Here's how the part is built. I have some questions about the finished solid (model axes, mm). Face numbers are marked on the shaded views. Give positions to 0.01 mm unless a question says otherwise; leave off trailing zeros. Loops run counter-clockwise (first coordinate to the right, second up) from the corner with the lowest first, then second, coordinate; pieces in that order, holes last. Notation, with made-up numbers: (78.5, -4.75) - (127.5, -4.75) arc R27 cw to (127.5, 25.25) - close; hole circle Ø3 at (30.5, 40.5). An arc over 180 degrees is marked (long way). Use a Markdown table: item, result.
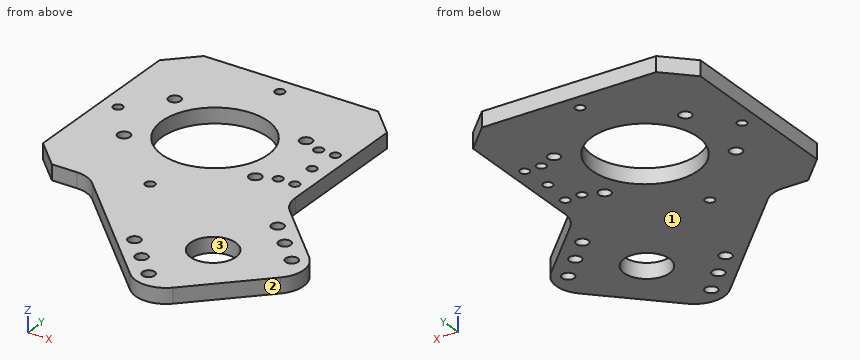
Autodesk Inventor part; units mm, degrees
ref_plane "YZ Plane" through (0, 0, 0) normal (1, 0, 0) x (0, 1, 0)
ref_plane "XZ Plane" through (0, 0, 0) normal (0, 1, 0) x (-1, 0, 0)
ref_plane "XY Plane" through (0, 0, 0) normal (0, 0, 1) x (1, 0, 0)
sketch "Sketch1" plane through (0, 0, 0) normal (0, 0, 1) x (1, 0, 0)
  line L0 (-47.625, -47.625) -> (47.625, -47.625)
  line L1 (47.625, -47.625) -> (47.625, 47.625)
  line L2 (47.625, 47.625) -> (-47.625, 47.625)
  line L3 (-47.625, 47.625) -> (-47.625, -47.625)
  line L4 (-47.625, -47.625) -> (47.625, 47.625) construction
  line L5 (47.625, -47.625) -> (-47.625, 47.625) construction
  point P0 (0, 0)
  dimension "width" = 95.25
  dimension "length" = 95.25
extrude "Extrusion1" add sketch "Sketch1" along normal mid plane 6.35
sketch "Sketch2" plane through (0, 0, 3.175) normal (0, 0, 1) x (1, 0, 0)
  circle A0 centre (0, 0) radius 35
  circle A1 centre (0, 0) radius 60 construction
  circle A2 centre (0, 0) radius 40.64 construction
  point P0 (0, 40.64)
  point P1 (-40.64, 0)
  point P2 (0, -40.64)
  point P3 (40.64, 0)
  dimension "d74" = 81.28
  dimension "d5" = 120
  dimension "d73" = 70
  dimension "d77" = 360
hole "Hole1" at (0, 40.64, 3.175) at (-40.64, 0, 3.175) at (0, -40.64, 3.175) at (40.64, 0, 3.175) direction (0, 0, -1) diameter 3.9624 end through all
sketch "Sketch3" plane through (0, 0, 3.175) normal (0, 0, 1) x (1, 0, 0)
  circle A0 centre (0, 0) radius 31.75 construction
  point P0 (0, 31.75)
  point P1 (-27.4963, 15.875)
  point P2 (-27.4963, -15.875)
  point P3 (0, -31.75)
  point P4 (27.4963, -15.875)
  point P5 (27.4963, 15.875)
  dimension "d17" = 63.5
  dimension "d20" = 360
hole "Hole2" at (-27.4963, 15.875, 3.175) at (-27.4963, -15.875, 3.175) at (27.4963, -15.875, 3.175) at (27.4963, 15.875, 3.175) direction (0, 0, -1) diameter 5.1054 end through all
sketch "Sketch4" plane through (0, 0, 3.175) normal (0, 0, 1) x (1, 0, 0)
  circle A0 centre (0, 0) radius 22.225
  dimension "d30" = 44.45
extrude "Extrusion2" cut sketch "Sketch4" against normal through all
sketch "Sketch5" plane through (0, 0, 3.175) normal (0, 0, 1) x (1, 0, 0)
  circle A0 centre (0, 0) radius 64 construction
  circle A1 centre (45.021, -68.5355) radius 18 construction
  line L0 (95.821, 47.9105) -> (95.821, -47.9105) construction
  line L1 (54.0013, -41.5947) -> (18.0802, -77.5157) construction
  line L2 (18.0802, -77.5157) -> (27.0605, -86.496) construction
  line L3 (36.0407, -59.5552) -> (45.021, -68.5355) construction
  line L4 (-47.625, -47.625) -> (47.625, -47.625) construction
  line L5 (-20.7907, -47.625) -> (39.7884, -108.2042)
  line L6 (39.7884, -108.2042) -> (84.6897, -63.3029)
  line L7 (84.6897, -63.3029) -> (47.625, -26.2382)
  line L8 (47.625, -47.625) -> (47.625, 47.625) construction
  line L9 (-20.7907, -47.625) -> (47.625, -47.625)
  line L10 (47.625, -47.625) -> (47.625, -26.2382)
  circle A2 centre (45.021, -68.5355) radius 9.525
  point P0 (95.821, 0)
  point P1 (27.0605, -86.496)
  point P2 (36.0407, -95.4762)
  point P3 (62.9815, -50.5749)
  point P4 (62.9815, -50.5749)
  point P5 (71.9618, -59.5552)
  point P6 (-22.225, -47.625)
  dimension "d33" = 128
  dimension "d34" = 36
  dimension "d35" = 95.821
  dimension "d36" = 95.821
  dimension "d37" = 50.8
  dimension "d38" = 12.7
  dimension "d39" = 12.7
  dimension "d42" = 12.7
  dimension "d47" = 45
  dimension "d48" = 50.8
  dimension "d49" = 6.35
  dimension "d50" = 24.35
  dimension "d51" = 6.35
  dimension "d55" = 19.05
  dimension "d64" = 45
extrude "Extrusion3" add sketch "Sketch5" against normal up to surface (6.35 mm away)
hole "Hole3" at (18.0802, -77.5157, 3.175) at (27.0605, -86.496, 3.175) at (36.0407, -95.4762, 3.175) at (54.0013, -41.5947, 3.175) at (71.9618, -59.5552, 3.175) at (62.9815, -50.5749, 3.175) direction (0, 0, -1) diameter 5.1054 end through all
fillet "Fillet2" radius 12.7 4 edges at (47.625, -26.2382, 0) (-20.7907, -47.625, 0) (39.7884, -108.2042, 0) (84.6897, -63.3029, 0)
sketch "Sketch7" plane through (0, 0, 3.175) normal (0, 0, 1) x (1, 0, 0)
  circle A0 centre (0, 0) radius 60 construction
  circle A1 centre (71.9618, -59.5552) radius 2.5527 construction
  circle A2 centre (36.0407, -95.4762) radius 2.5527 construction
  circle A3 centre (18.0802, -77.5157) radius 2.5527 construction
  circle A4 centre (27.0605, -86.496) radius 2.5527 construction
  circle A5 centre (54.0013, -41.5947) radius 2.5527 construction
  circle A6 centre (62.9815, -50.5749) radius 2.5527 construction
  circle A7 centre (45.021, -68.5355) radius 9.525 construction
  circle A8 centre (0, 0) radius 22.225 construction
  circle A9 centre (27.4963, -15.875) radius 2.5527 construction
  circle A10 centre (-27.4963, -15.875) radius 2.5527 construction
  circle A11 centre (-27.4963, 15.875) radius 2.5527 construction
  circle A12 centre (27.4963, 15.875) radius 2.5527 construction
  arc A13 (75.7094, -72.2831) -> (75.7094, -54.3226) centre (66.7292, -63.3029) ccw construction
  line L0 (75.7094, -54.3226) -> (51.3447, -29.9579) construction
  arc A14 (47.625, -20.9777) -> (51.3447, -29.9579) centre (60.325, -20.9777) ccw construction
  line L1 (47.625, -20.9777) -> (47.625, 47.625) construction
  line L2 (47.625, 47.625) -> (-47.625, 47.625) construction
  line L3 (-47.625, 47.625) -> (-47.625, -47.625) construction
  line L4 (-47.625, -47.625) -> (-26.0513, -47.625) construction
  arc A15 (-17.071, -51.3447) -> (-26.0513, -47.625) centre (-26.0513, -60.325) ccw construction
  line L5 (-17.071, -51.3447) -> (30.8082, -99.2239) construction
  arc A16 (30.8082, -99.2239) -> (48.7687, -99.2239) centre (39.7884, -90.2436) ccw construction
  line L6 (48.7687, -99.2239) -> (75.7094, -72.2831) construction
  line L7 (-47.625, 47.625) -> (47.625, 47.625) construction
  line L8 (-36.4946, 47.625) -> (-47.625, 47.625)
  line L9 (-47.625, 47.625) -> (-47.625, 36.4946)
  line L10 (-47.625, -47.625) -> (-47.625, 47.625) construction
  line L11 (36.4946, 47.625) -> (47.625, 47.625)
  line L12 (47.625, 47.625) -> (47.625, 36.4946)
  line L13 (47.625, 47.625) -> (47.625, -20.9777) construction
  line L14 (-47.625, -36.4946) -> (-47.625, -47.625)
  line L15 (-26.0513, -47.625) -> (-47.625, -47.625) construction
  line L16 (-47.625, -47.625) -> (-36.4946, -47.625)
  line L17 (-47.625, -36.4946) -> (-36.4946, -47.625)
  line L18 (36.4946, 47.625) -> (47.625, 36.4946)
  line L19 (-36.4946, 47.625) -> (-47.625, 36.4946)
  dimension "d68" = 120
extrude "Extrusion5" cut sketch "Sketch7" against normal through all
sketch "Sketch8" plane through (0, 0, -3.175) normal (0, 0, -1) x (-1, 0, 0)
  line L0 (-34.925, -12.7) -> (-34.925, 12.7) construction
  circle A0 centre (-40.64, 0) radius 1.9812 construction
  circle A1 centre (40.64, 0) radius 1.9812 construction
  circle A2 centre (0, 40.64) radius 1.9812 construction
  circle A3 centre (0, -40.64) radius 1.9812 construction
  circle A4 centre (-27.4963, 15.875) radius 2.5527 construction
  circle A5 centre (27.4963, -15.875) radius 2.5527 construction
  circle A6 centre (27.4963, 15.875) radius 2.5527 construction
  circle A7 centre (-27.4963, -15.875) radius 2.5527 construction
  circle A8 centre (0, 0) radius 22.225 construction
  circle A9 centre (-45.021, -68.5355) radius 9.525 construction
  circle A10 centre (-62.9815, -50.5749) radius 2.5527 construction
  circle A11 centre (-54.0013, -41.5947) radius 2.5527 construction
  circle A12 centre (-27.0605, -86.496) radius 2.5527 construction
  circle A13 centre (-18.0802, -77.5157) radius 2.5527 construction
  circle A14 centre (-36.0407, -95.4762) radius 2.5527 construction
  circle A15 centre (-71.9618, -59.5552) radius 2.5527 construction
  line L1 (36.4946, -47.625) -> (47.625, -36.4946) construction
  line L2 (47.625, -36.4946) -> (47.625, 36.4946) construction
  line L3 (47.625, 36.4946) -> (36.4946, 47.625) construction
  line L4 (36.4946, 47.625) -> (-36.4946, 47.625) construction
  line L5 (-36.4946, 47.625) -> (-47.625, 36.4946) construction
  line L6 (-47.625, 36.4946) -> (-47.625, -20.9777) construction
  arc A16 (-51.3447, -29.9579) -> (-47.625, -20.9777) centre (-60.325, -20.9777) ccw construction
  line L7 (-75.7094, -54.3226) -> (-51.3447, -29.9579) construction
  arc A17 (-75.7094, -54.3226) -> (-75.7094, -72.2831) centre (-66.7292, -63.3029) ccw construction
  line L8 (-48.7687, -99.2239) -> (-75.7094, -72.2831) construction
  arc A18 (-48.7687, -99.2239) -> (-30.8082, -99.2239) centre (-39.7884, -90.2436) ccw construction
  line L9 (17.071, -51.3447) -> (-30.8082, -99.2239) construction
  arc A19 (26.0513, -47.625) -> (17.071, -51.3447) centre (26.0513, -60.325) ccw construction
  line L10 (26.0513, -47.625) -> (36.4946, -47.625) construction
  point P0 (-34.925, 0)
  dimension "d79" = 25.4
  dimension "d80" = 12.7
  dimension "d88" = 34.925
  dimension "d89" = 44.45
hole "Hole4" at (34.925, -12.7, -3.175) at (34.925, 12.7, -3.175) direction (0, 0, 1) diameter 3.9624 end through all
sketch "Sketch9" plane through (0, 0, -3.175) normal (0, 0, -1) x (-1, 0, 0)
  circle A0 centre (-34.925, -12.7) radius 1.9812 construction
  circle A1 centre (-34.925, 12.7) radius 1.9812 construction
  arc A2 (-51.3447, -29.9579) -> (-47.625, -20.9777) centre (-60.325, -20.9777) ccw construction
  line L0 (-47.625, -20.9777) -> (-47.625, 36.4946) construction
  line L1 (-47.625, 36.4946) -> (-36.4946, 47.625) construction
  line L2 (-36.4946, 47.625) -> (36.4946, 47.625) construction
  line L3 (36.4946, 47.625) -> (47.625, 36.4946) construction
  line L4 (47.625, 36.4946) -> (47.625, -36.4946) construction
  line L5 (47.625, -36.4946) -> (36.4946, -47.625) construction
  line L6 (36.4946, -47.625) -> (26.0513, -47.625) construction
  arc A3 (26.0513, -47.625) -> (17.071, -51.3447) centre (26.0513, -60.325) ccw construction
  line L7 (17.071, -51.3447) -> (-30.8082, -99.2239) construction
  arc A4 (-48.7687, -99.2239) -> (-30.8082, -99.2239) centre (-39.7884, -90.2436) ccw construction
  line L8 (-48.7687, -99.2239) -> (-75.7094, -72.2831) construction
  arc A5 (-75.7094, -54.3226) -> (-75.7094, -72.2831) centre (-66.7292, -63.3029) ccw construction
  line L9 (-75.7094, -54.3226) -> (-51.3447, -29.9579) construction
  circle A6 centre (-71.9618, -59.5552) radius 2.5527 construction
  circle A7 centre (-36.0407, -95.4762) radius 2.5527 construction
  circle A8 centre (-18.0802, -77.5157) radius 2.5527 construction
  circle A9 centre (-27.0605, -86.496) radius 2.5527 construction
  circle A10 centre (-54.0013, -41.5947) radius 2.5527 construction
  circle A11 centre (-62.9815, -50.5749) radius 2.5527 construction
  circle A12 centre (-45.021, -68.5355) radius 9.525 construction
  circle A13 centre (0, 0) radius 22.225 construction
  circle A14 centre (-27.4963, -15.875) radius 2.5527 construction
  circle A15 centre (27.4963, 15.875) radius 2.5527 construction
  circle A16 centre (27.4963, -15.875) radius 2.5527 construction
  circle A17 centre (-27.4963, 15.875) radius 2.5527 construction
  circle A18 centre (0, -40.64) radius 1.9812 construction
  circle A19 centre (0, 40.64) radius 1.9812 construction
  circle A20 centre (40.64, 0) radius 1.9812 construction
  circle A21 centre (-40.64, 0) radius 1.9812 construction
  circle A22 centre (-41.91, -12.7) radius 2.5527 construction
  point P0 (-41.91, 12.7)
  dimension "d90" = 5.715
  dimension "d91" = 5.1054
hole "Hole5" at (41.91, -12.7, -3.175) at (41.91, 12.7, -3.175) direction (0, 0, 1) diameter 3.9624 end through all
equation "\"d36\" = d35"
equation "\"d39\" = d38"
equation "\"d50\" = 0.5 * d34 + d49"
equation "\"d64\" = d47"
equation "\"d63\" = d29"
properties part number "GP6-004" material "Aluminum 6061"
(1) Suppose I cut it at D-D on y = -40.64. Write out the boundary of the cut face in (x, z) (3 decimals), plus the area to 3 significant figures.
A:
| item | result |
|---|---|
| outline | (-43.48, -3.175) - (-1.981, -3.175) - (-1.981, 3.175) - (-43.48, 3.175) - close; (1.981, -3.175) - (51.634, -3.175) - (51.634, 3.175) - (1.981, 3.175) - close; (56.369, -3.175) - (62.027, -3.175) - (62.027, 3.175) - (56.369, 3.175) - close |
| area | 615 mm2 |
(2) Suppose I cut it at C-C on z = 2. Count the separate pieces of the cut face and the enclosed holes in it, plus the area to 3 significant figures.
A:
| item | result |
|---|---|
| separate pieces | 1 |
| enclosed holes | 20 |
| area | 10,300 mm2 |
(3) We'd pull the mould along X, two halves only. Please class the marked faces 1, 2 and 3: pulls with the +X half, pulls with the -X half, needs draft (parallel to the pull), parting line crosses it, or undercut.
A:
| item | result |
|---|---|
| face 1 | needs draft |
| face 2 | pulls with the +X half |
| face 3 | undercut |
(4) If I drill on line 1 (Y direction, x = 41.91, z = -0.75); line 2 (Y direction, x = 40.64, z = 1.5); line 3 (X direction, y = -16, z = -2.5) (3 decimals), over which ranges is the centre line in solid material (lowest first)?
A:
| item | result |
|---|---|
| line 1 | -102.77 to -77.54, -59.53 to -14.68, -10.72 to -1.52, 1.52 to 10.72, 14.68 to 42.21 |
| line 2 | -102.92 to -76.99, -60.08 to -14.22, -11.18 to -1.98, 1.98 to 11.18, 14.22 to 43.48 |
| line 3 | -47.625 to -30.046, -24.947 to -15.426, 15.426 to 24.947, 30.046 to 47.625 |
(5) Will these pins go through, and if not, where does the flat tip stop? pin 1 (2 mm diameter, centred on x = -25.5, z = 2, fed in from -Y); pin 2 (3 mm diameter, centred on x = 0, y = 40.64, fed in from +Z); pin 3 (1 mm diameter, centred on y = -65, z = -0.5, fed in from +X); pin 4 (1 mm diameter, centred on x = -14, z = -1.5, fed in from -Y).
A:
| item | result |
|---|---|
| pin 1 | y = -47.72 |
| pin 2 | through |
| pin 3 | x = 79.37 |
| pin 4 | y = -54.92 |
(6) Suppose I cut it at A-A on x = 12. Write out the boundary of the cut face in (y, z) (3 decimals), plus the area to 3 significant figures.
A:
| item | result |
|---|---|
| outline | (-80.416, -3.175) - (-18.707, -3.175) - (-18.707, 3.175) - (-80.416, 3.175) - close; (18.707, -3.175) - (47.625, -3.175) - (47.625, 3.175) - (18.707, 3.175) - close |
| area | 575 mm2 |
(7) Suppose I cut it at B-B on y = 7.5. Write out the boundary of the cut face in (x, z) (3 decimals), plus the area to 3 significant figures.
A:
| item | result |
|---|---|
| outline | (-47.625, -3.175) - (-20.921, -3.175) - (-20.921, 3.175) - (-47.625, 3.175) - close; (20.921, -3.175) - (47.625, -3.175) - (47.625, 3.175) - (20.921, 3.175) - close |
| area | 339 mm2 |
